Verification items for this drawing (mm, ordinates from the low corner). A direction names the side the tool comes from. Round coordinates to 2 decimals unless told otherwise and drop trailing zeros. Loops run counter-clockwise (first coordinate to the right, second up) from the corner with the lowest first, then second, coordinate; pieces in that order, holes last. Notation, with made-up numbers: M 68,54.5 L 125,54.5 A14 cw 125,78.5 Z; hole C 81,10 d2. An arc over 180 degrees is marked long. Answer in a Markdown table with one row per item. Add a question column.
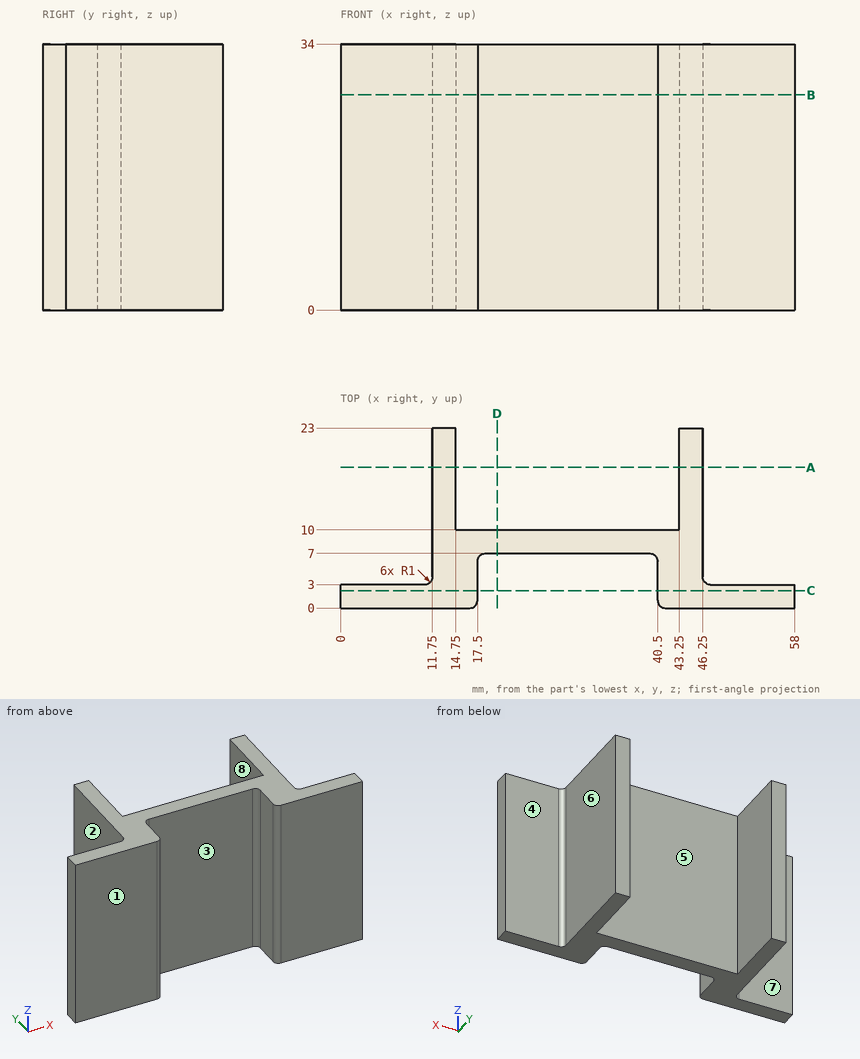
1) Draft check along X on the marked faces 6, 7 and 8. Enter one of: +X half, -X half, draft (parallel to the pull), parting line (faces both ways), or undercut.
2) Cross-section at B-B, the plane z = 27.5. Record the boundary of the cut face in (x, y), plus the area to 3 significant figures.
3) Set-up check for the marked faces 1, 2, 3, 4 and 5: record each of +Z, -Z, +X, -X, +Y, -Y from which the full face is reachable in a straight line by a thin tool's end or side.
4) Cross-section at C-C, the plane y = 2.25. Record the boundary of the cut face in (x, z), plus the area to 3 significant figures.
5) Thickness scan on L1, parallel to X at y = 18.25, z = 10; L2, parallel to X at y = 2, z = 22; L3, parallel to X at y = 8.75, z = 32.5. Record the ranges inside material, lowest first. Write a range as [from, to].
6) Go/stop test with flat-tipped pins: pin 1 (8.5 mm diameter, centred on x = 31.5, z = 10, fed in from +Y); pin 2 (12 mm diameter, centred on x = 51.5, z = 14, fed in from +Y); pin 3 (10.5 mm diameter, centred on y = 19.5, z = 10, fed in from +X); pin 4 (4 mm diameter, centred on y = 19, z = 10, fed in from -X). Record where each tip stops, or that it passes through.
7) Cross-section at D-D, the plane x = 20. Record the boundary of the cut face in (y, z), plus the area to 3 significant figures.
8) Cross-section at A-A, the plane y = 18. Record the boundary of the cut face in (x, z), plus the area to 3 significant figures.
Worked answers:
| question | item | result |
|---|---|---|
| 1 | face 6 | +X half |
| 1 | face 7 | draft |
| 1 | face 8 | undercut |
| 2 | outline | M 0,0 L 16.5,0 A1 ccw 17.5,1 L 17.5,6 A1 cw 18.5,7 L 39.5,7 A1 cw 40.5,6 L 40.5,1 A1 ccw 41.5,0 L 58,0 L 58,3 L 47.25,3 A1 cw 46.25,4 L 46.25,23 L 43.25,23 L 43.25,10 L 14.75,10 L 14.75,23 L 11.75,23 L 11.75,4 A1 cw 10.75,3 L 0,3 Z |
| 2 | area | 333 mm2 |
| 3 | face 1 | +Z, -Z, +X, -X, -Y |
| 3 | face 2 | +Z, -Z, -X, +Y |
| 3 | face 3 | +Z, -Z, -Y |
| 3 | face 4 | +Z, -Z, +X, +Y |
| 3 | face 5 | +Z, -Z, +Y |
| 4 | outline | M 0,0 L 17.5,0 L 17.5,34 L 0,34 Z; M 40.5,0 L 58,0 L 58,34 L 40.5,34 Z |
| 4 | area | 1,190 mm2 |
| 5 | L1 | x = [11.75, 14.75], [43.25, 46.25] |
| 5 | L2 | x = [0, 17.5], [40.5, 58] |
| 5 | L3 | x = [11.75, 46.25] |
| 6 | pin 1 | stops at y = 10 |
| 6 | pin 2 | stops at y = 23 |
| 6 | pin 3 | stops at x = 46.25 |
| 6 | pin 4 | stops at x = 11.75 |
| 7 | outline | M 7,0 L 10,0 L 10,34 L 7,34 Z |
| 7 | area | 102 mm2 |
| 8 | outline | M 11.75,0 L 14.75,0 L 14.75,34 L 11.75,34 Z; M 43.25,0 L 46.25,0 L 46.25,34 L 43.25,34 Z |
| 8 | area | 204 mm2 |
